Design review of the part shown in the three views and the two pictorial views. Dimensions are in mm from the part's minimum x, y and z. Round coordinates to 2 decimals unless told otherwise and drop trailing zeros. Loops run counter-clockwise (first coordinate to the right, second up) from the corner with the lowest first, then second, coordinate; pieces in that order, holes last. Notation, with made-up numbers: M -16.75,26.5 L 38.25,26.5 A16 cw 38.25,35.5 Z; hole C -23,-8 d11. An arc over 180 degrees is marked long. One line per question, with ' | ' between items. Start each with the question number.
1) We need section B-B (x = 7). Give the boundary of the cut face in (y, z).
2) We need section D-D (y = 80). Give the boundary of the cut face in (x, z).
3) We need section C-C (y = 23). Give the boundary of the cut face in (x, z).
4) Mouldability with a two-part tool opening along Y and no side actions: class the marked faces 1, 2, 3 and 4 as pulls with the +Y half, pulls with the -Y half, needs draft (parallel to the pull), parting line crosses it, or undercut.
5) For pin 1 Ø4 at (y, z) = (74.5, 2.5) entering from -X; pin 2 Ø1 at (y, z) = (61, 5) entering from +X; pin 3 Ø3.5 at (y, z) = (96.5, 5) entering from +X, all flat-tipped, find the tip position at first contact; note any pin that passes through.
6) For probe 1 along Y at (x, z) = (15, 6.95); probe 2 along Y at (x, z) = (7, 6.6); probe 3 along X at (y, z) = (74.5, 4), list the stretches that pass through material, from the lowest coordinate up. Write a range as from..to.
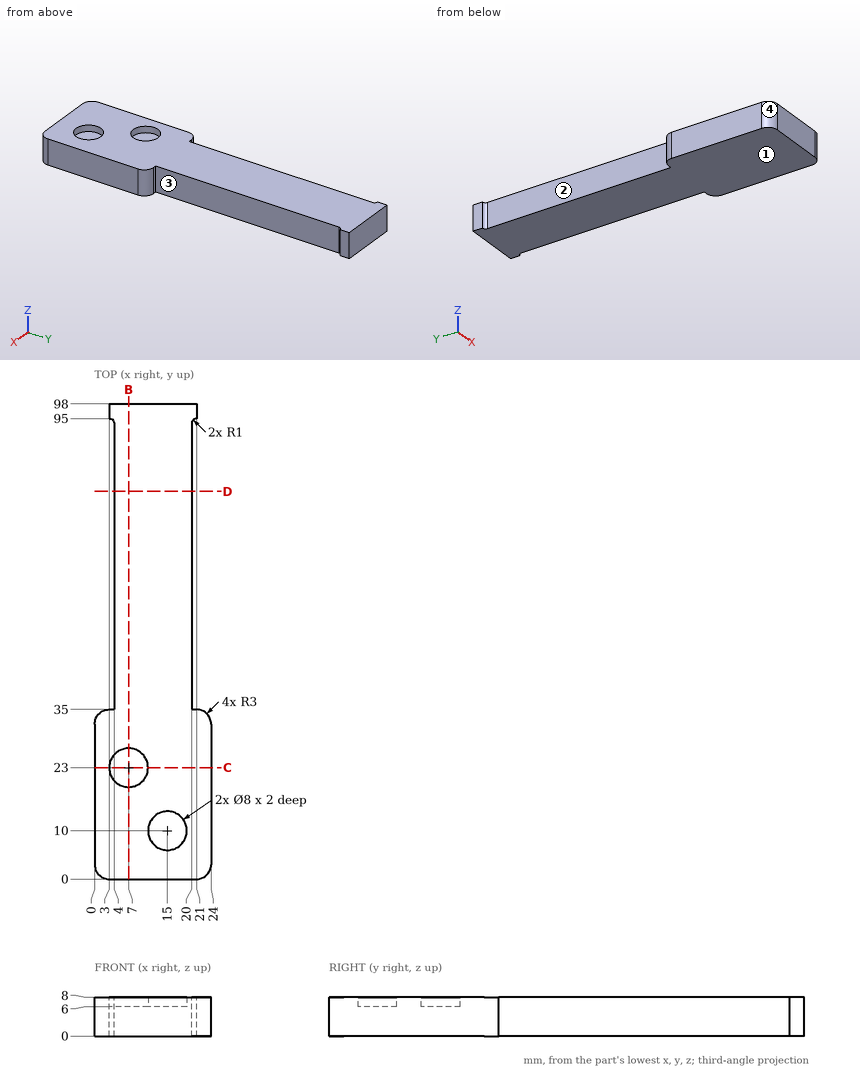
Answers below:
1) outline: M 0,0 L 98,0 L 98,8 L 27,8 L 27,6 L 19,6 L 19,8 L 0,8 Z
2) outline: M 4,0 L 20,0 L 20,8 L 4,8 Z
3) outline: M 0,0 L 24,0 L 24,8 L 11,8 L 11,6 L 3,6 L 3,8 L 0,8 Z
4) face 1: needs draft | face 2: undercut | face 3: undercut | face 4: pulls with the -Y half
5) pin 1: x = 4 | pin 2: x = 20 | pin 3: x = 21
6) probe 1: 0..6, 14..98 | probe 2: 0..19, 27..98 | probe 3: 4..20
